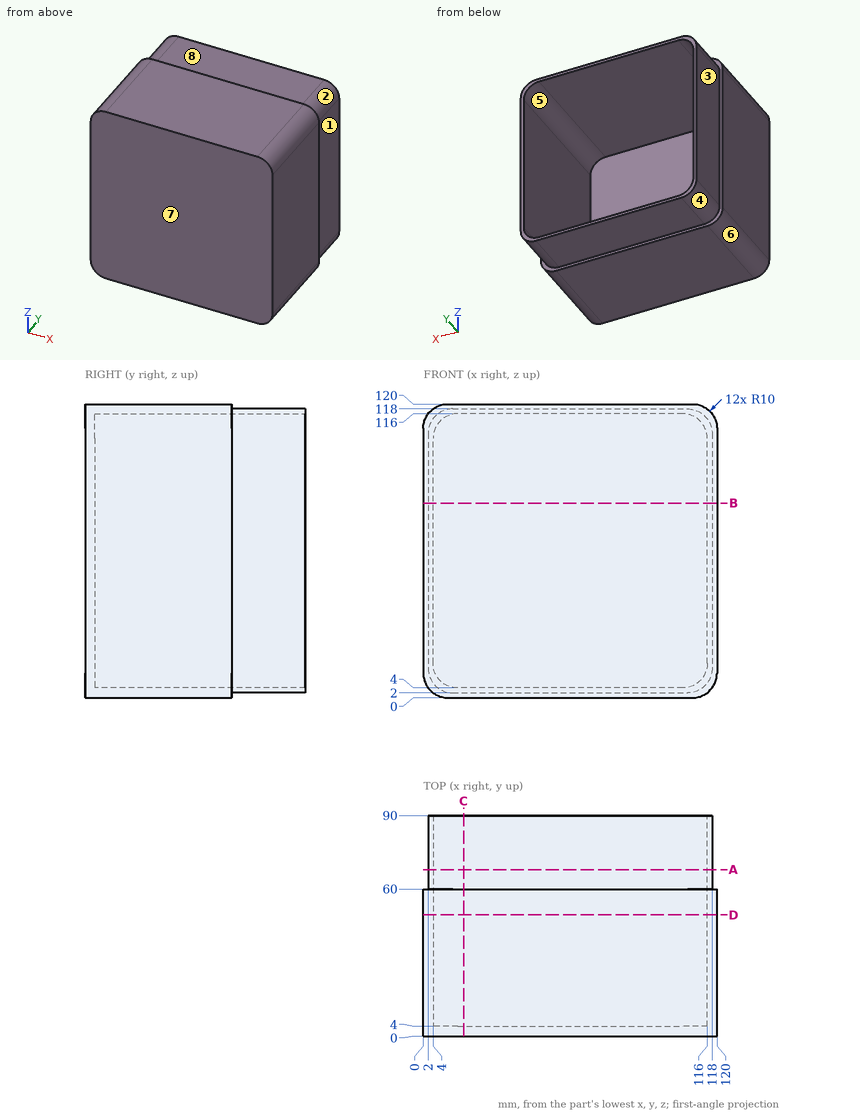
Design review of the part shown in the three views and the two pictorial views. Dimensions are in mm from the part's minimum x, y and z. A direction names the side the tool comes from. Round coordinates to 2 decimals unless told otherwise and drop trailing zeros. Loops run counter-clockwise (first coordinate to the right, second up) from the corner with the lowest first, then second, coordinate; pieces in that order, holes last. Notation, with made-up numbers: (12.5, 62) - (45.5, 62) arc R13 ccw to (45.5, 76) - close; hole circle Ø8 at (21, -22). An arc over 180 degrees is marked (long way). One line per item, written item: value. Start each with the question number.
Item 1: For L1, parallel to Z at x = 38, y = 47; L2, parallel to X at y = 79.5, z = 14.5, list the stretches that pass through material, from the lowest coordinate up.
Item 2: For the marked faces 1, 2, 3 and 4, list the 3-axis set-ups (+Z, -Z, +X, -X, +Y, -Y) from which the entire face can be reached by the end or side of a thin tool; tool diameter is ignored.
Item 3: Take a section at A-A (y = 68). Give the boundary of the cut face in (x, z).
Item 4: Clearance check with flat-ended pins moving along their axes: pin 1 Ø10 at (y, z) = (44.5, 27.5) entering from -X; pin 2 Ø15 at (y, z) = (74.5, 40) entering from +X; pin 3 Ø9 at (x, y) = (58.5, 77) entering from -Z; pin 4 Ø9 at (x, y) = (68.5, 67.5) entering from +Z. State where each tip first meets the part, or that it passes through.
Item 5: Take a section at C-C (x = 16.5). Give the boundary of the cut face in (y, z).
Item 6: The part is to be moulded in two halves that separate along Z. For the marked faces 5, 6, 7 and 8, say which applies: +Z half, -Z half, draft (parallel to the pull), parting line (faces both ways), or undercut.
Item 7: Take a section at D-D (y = 49.5). Give the boundary of the cut face in (x, z), plus the area to 3 significant figures.
Item 8: Take a section at B-B (z = 79.5). Give the boundary of the cut face in (x, y), plus the area to 3 significant figures.
Answer below:
1. L1: z = 0 to 4, 116 to 120
1. L2: x = 2 to 4, 116 to 118
2. face 1: +Z, -Z, +X, +Y
2. face 2: +Z, +X, +Y
2. face 3: +Z, -Z, -X, +Y
2. face 4: -Z, -X, +Y
3. outline: (2, 12) arc R10 ccw to (12, 2) - (108, 2) arc R10 ccw to (118, 12) - (118, 108) arc R10 ccw to (108, 118) - (12, 118) arc R10 ccw to (2, 108) - close; hole (4, 14) arc R10 ccw to (14, 4) - (106, 4) arc R10 ccw to (116, 14) - (116, 106) arc R10 ccw to (106, 116) - (14, 116) arc R10 ccw to (4, 106) - close
4. pin 1: stops at x = 0
4. pin 2: stops at x = 118
4. pin 3: stops at z = 2
4. pin 4: stops at z = 118
5. outline: (0, 0) - (60, 0) - (60, 2) - (90, 2) - (90, 4) - (4, 4) - (4, 116) - (90, 116) - (90, 118) - (60, 118) - (60, 120) - (0, 120) - close
6. face 5: undercut
6. face 6: -Z half
6. face 7: draft
6. face 8: +Z half
7. outline: (0, 10) arc R10 ccw to (10, 0) - (110, 0) arc R10 ccw to (120, 10) - (120, 110) arc R10 ccw to (110, 120) - (10, 120) arc R10 ccw to (0, 110) - close; hole (4, 14) arc R10 ccw to (14, 4) - (106, 4) arc R10 ccw to (116, 14) - (116, 106) arc R10 ccw to (106, 116) - (14, 116) arc R10 ccw to (4, 106) - close
7. area: 1,860 mm2
8. outline: (0, 0) - (120, 0) - (120, 60) - (118, 60) - (118, 90) - (116, 90) - (116, 4) - (4, 4) - (4, 90) - (2, 90) - (2, 60) - (0, 60) - close
8. area: 1,050 mm2
